```python
from build123d import *

# Parameters (mm, degrees)
SKETCH1_R           = 2.1
BOSS_EXTRUDE1_DEPTH = 707


with BuildPart() as part:
    # Sketch1 → Boss-Extrude1 (new body)
    with BuildSketch(Plane(origin=(0, 0, 0), x_dir=(0, 0, -1), z_dir=(1, 0, 0))):
        with BuildLine():
            Line((-10, 7), (-10, -7))
            Line((-10, -7), (-8, -7))
            Line((-8, -7), (-8, -4))
            Line((-8, -4), (-7.060660172, -4))
            Line((-7.060660172, -4), (-4, -7.060660172))
            Line((-4, -7.060660172), (-4, -12.939339828))
            Line((-4, -12.939339828), (-7.060660172, -16))
            Line((-7.060660172, -16), (-8, -16))
            Line((-8, -16), (-8, -13))
            Line((-8, -13), (-10, -13))
            Line((-10, -13), (-10, -19))
            ThreePointArc((-10, -19), (-9.948683298, -19.316227766), (-9.8, -19.6))
            Line((-9.8, -19.6), (-3, -19.6))
            Line((-3, -19.6), (-3, -18))
            Line((-3, -18), (-6, -18))
            Line((-6, -18), (-6, -17.060660172))
            Line((-6, -17.060660172), (-2.939339828, -14))
            Line((-2.939339828, -14), (2.939339828, -14))
            Line((2.939339828, -14), (6, -17.060660172))
            Line((6, -17.060660172), (6, -18))
            Line((6, -18), (3, -18))
            Line((3, -18), (3, -19.6))
            Line((3, -19.6), (9.8, -19.6))
            ThreePointArc((9.8, -19.6), (9.948683298, -19.316227766), (10, -19))
            Line((10, -19), (10, -13))
            Line((10, -13), (8, -13))
            Line((8, -13), (8, -16))
            Line((8, -16), (7.060660172, -16))
            Line((7.060660172, -16), (4, -12.939339828))
            Line((4, -12.939339828), (4, -7.060660172))
            Line((4, -7.060660172), (7.060660172, -4))
            Line((7.060660172, -4), (8, -4))
            Line((8, -4), (8, -7))
            Line((8, -7), (10, -7))
            Line((10, -7), (10, 7))
            Line((10, 7), (8, 7))
            Line((8, 7), (8, 4))
            Line((8, 4), (7.060660172, 4))
            Line((7.060660172, 4), (4, 7.060660172))
            Line((4, 7.060660172), (4, 12.939339828))
            Line((4, 12.939339828), (7.060660172, 16))
            Line((7.060660172, 16), (8, 16))
            Line((8, 16), (8, 13))
            Line((8, 13), (10, 13))
            Line((10, 13), (10, 19))
            ThreePointArc((10, 19), (9.948683298, 19.316227766), (9.8, 19.6))
            Line((9.8, 19.6), (3, 19.6))
            Line((3, 19.6), (3, 18))
            Line((3, 18), (6, 18))
            Line((6, 18), (6, 17.060660172))
            Line((6, 17.060660172), (2.939339828, 14))
            Line((2.939339828, 14), (-2.939339828, 14))
            Line((-2.939339828, 14), (-6, 17.060660172))
            Line((-6, 17.060660172), (-6, 18))
            Line((-6, 18), (-3, 18))
            Line((-3, 18), (-3, 19.6))
            Line((-3, 19.6), (-9.8, 19.6))
            ThreePointArc((-9.8, 19.6), (-9.948683298, 19.316227766), (-10, 19))
            Line((-10, 19), (-10, 13))
            Line((-10, 13), (-8, 13))
            Line((-8, 13), (-8, 16))
            Line((-8, 16), (-7.060660172, 16))
            Line((-7.060660172, 16), (-4, 12.939339828))
            Line((-4, 12.939339828), (-4, 7.060660172))
            Line((-4, 7.060660172), (-7.060660172, 4))
            Line((-7.060660172, 4), (-8, 4))
            Line((-8, 4), (-8, 7))
            Line((-8, 7), (-10, 7))
        make_face()
        with Locations((0, 10)):
            Circle(SKETCH1_R, mode=Mode.SUBTRACT)
        with Locations((0, -10)):
            Circle(SKETCH1_R, mode=Mode.SUBTRACT)
        with BuildLine():
            Line((-8, 1.7), (-8, -1.7))
            ThreePointArc((-8, -1.7), (-7.912132034, -1.912132034), (-7.7, -2))
            Line((-7.7, -2), (-7.063603897, -2))
            ThreePointArc((-7.063603897, -2), (-6.948798867, -2.02283614), (-6.851471863, -2.087867966))
            Line((-6.851471863, -2.087867966), (-2.939339828, -6))
            Line((-2.939339828, -6), (2.939339828, -6))
            Line((2.939339828, -6), (6.851471863, -2.087867966))
            ThreePointArc((6.851471863, -2.087867966), (6.948798867, -2.02283614), (7.063603897, -2))
            Line((7.063603897, -2), (7.7, -2))
            ThreePointArc((7.7, -2), (7.912132034, -1.912132034), (8, -1.7))
            Line((8, -1.7), (8, 1.7))
            ThreePointArc((8, 1.7), (7.912132034, 1.912132034), (7.7, 2))
            Line((7.7, 2), (7.063603897, 2))
            ThreePointArc((7.063603897, 2), (6.948798867, 2.02283614), (6.851471863, 2.087867966))
            Line((6.851471863, 2.087867966), (2.939339828, 6))
            Line((2.939339828, 6), (-2.939339828, 6))
            Line((-2.939339828, 6), (-6.851471863, 2.087867966))
            ThreePointArc((-6.851471863, 2.087867966), (-6.948798867, 2.02283614), (-7.063603897, 2))
            Line((-7.063603897, 2), (-7.7, 2))
            ThreePointArc((-7.7, 2), (-7.912132034, 1.912132034), (-8, 1.7))
        make_face(mode=Mode.SUBTRACT)
    extrude(amount=BOSS_EXTRUDE1_DEPTH)


solid = part.part
```
Input: part model. Units: mm. Frame: model coordinates. Give positions to 0.01 mm unless a question says otherwise; leave off trailing zeros. Write item = value, one per line. Start each with the question number.
1. First-contact query: pin 1 Ø1.8 at (x, z) = (190.5, -1.5) entering from -Y; pin 2 Ø3 at (x, y) = (113.5, -9.5) entering from -Z. Flat tips, straight axial feed; report the tip coordinate or a pass-through.
2. Ray query, L1, parallel to Y at x = 392, z = 0; L2, parallel to Y at x = 143.5, z = 0.5; L3, parallel to Y at x = 318, z = 9. Return the intervals inside material, ascending.
3. Section query A-A, the plane x = 162. Count the separate pieces of the cut face and the enclosed holes in it, then the cut area to 3 significant figures.
Check sheet entries:
q1.pin_1 = -14
q1.pin_2 = -4
q2.L1 = -14 to -12.1, -7.9 to -6, 6 to 7.9, 12.1 to 14
q2.L2 = -14 to -12.04, -7.96 to -6, 6 to 7.96, 12.04 to 14
q2.L3 = -19.6 to -13, -7 to 7, 13 to 19.6
q3.separate_pieces = 1
q3.enclosed_holes = 3
q3.area = 314 mm2
